Read the model definition and answer for the solid it produces. Units are mm, in the model's axes. Face numbers are marked on the shaded views. A direction names the side the tool comes from. Coordinates: 2 decimals unless noted, no trailing zeros. Loops run counter-clockwise (first coordinate to the right, second up) from the corner with the lowest first, then second, coordinate; pieces in that order, holes last. Notation, with made-up numbers: M 76,15.25 L 97,15.25 A14 ccw 97,19.25 Z; hole C 41.25,-38.75 d5. An arc over 180 degrees is marked long. One line per item, written item: value. Start each with the question number.
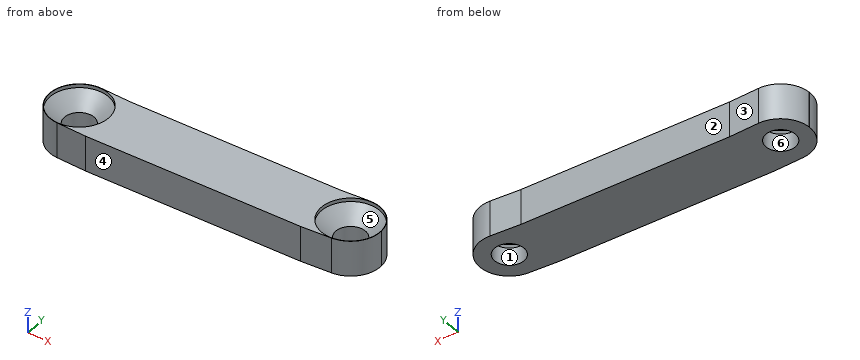
```python
from build123d import *

# Parameters (mm, degrees)
SKETCH1_R                                      = 1.25
BOSS_EXTRUDE1_DEPTH                            = 3
FILLET1_R                                      = 2.5
CSK_FOR_M2_5_FLAT_HEAD_MACHINE_SCREW2_AT_COUNT = 2
CSK_FOR_M2_5_FLAT_HEAD_MACHINE_SCREW2_AT_PITCH = 22.827023493


with BuildPart() as part:
    # Sketch1 → Boss-Extrude1 (new body)
    with BuildSketch(Plane.XY):
        Polygon((-14.040925474, -24.298454927), (-9.0477778, -24.560134708), (9.0477778, -24.560134708), (14.040925474, -24.298454927), (13.778886578, -19.298454927), (8.785738904, -19.560134708), (-8.785738904, -19.560134708), (-13.778886578, -19.298454927), align=None)
        with Locations((11.413511747, -21.93272098)):
            Circle(SKETCH1_R, mode=Mode.SUBTRACT)
        with Locations((-11.413511747, -21.93272098)):
            Circle(SKETCH1_R, mode=Mode.SUBTRACT)
    extrude(amount=BOSS_EXTRUDE1_DEPTH)

    # Fillet1
    fillet1_edges = [part.edges().sort_by_distance(p)[0] for p in [
        (-9.0477778, -24.560134708, 1.5),
        (-14.040925474, -24.298454927, 1.5),
        (-13.778886578, -19.298454927, 1.5),
        (-8.785738904, -19.560134708, 1.5),
        (8.785738904, -19.560134708, 1.5),
        (13.778886578, -19.298454927, 1.5),
        (14.040925474, -24.298454927, 1.5),
        (9.0477778, -24.560134708, 1.5),
    ]]
    fillet(fillet1_edges, radius=FILLET1_R)

    # Sketch5 → CSK for M2.5 Flat Head Machine Screw2 (revolve, cut)
    with BuildSketch(Plane(origin=(-11.413511747, -21.93272098, 3), x_dir=(0, -1, 0), z_dir=(1, 0, 0))):
        Polygon((0, 0), (0, 5.751075774), (1.25, 5), (1.25, 1.525), (2.475, 0.3), (2.475, 0), align=None)
    csk_for_m2_5_flat_head_machine_screw2 = revolve(axis=Axis((-11.413511747, -21.93272098, 9.35), (0, 0, -1)), mode=Mode.SUBTRACT)

    # CSK for M2.5 Flat Head Machine Screw2 at: CSK for M2.5 Flat Head Machine Screw2 ×2
    with Locations(*[(i * CSK_FOR_M2_5_FLAT_HEAD_MACHINE_SCREW2_AT_PITCH, 0, 0) for i in range(1, CSK_FOR_M2_5_FLAT_HEAD_MACHINE_SCREW2_AT_COUNT)]):
        add(csk_for_m2_5_flat_head_machine_screw2, mode=Mode.SUBTRACT)


solid = part.part
```
1) Section C-C (y = -22.4) is taken. Count the separate pieces of the cut face and the enclosed holes in it, then the cut area to 3 significant figures.
2) A flat-ended cylindrical pin translates along its axis: pin 1 (1.5 mm diameter, centred on x = 4.5, z = 1.5, fed in from +Y). Find the tip coordinate at first contact, or state that the pin passes through.
3) Section A-A (z = 2.1) is taken. Determine the outline of the cut face in (x, y) (3 decimals), then the cut area to 3 significant figures.
4) Consider line 1 along X through (y, z) = (-21.05, 1.65); line 2 along X through (y, z) = (-20.05, 2.6); line 3 along Y through (x, z) = (-3.5, 0.4). Determine where each line is inside the solid, lowest interval first.
5) For a pull along Y with two mould halves and no side action, classify the marked faces 3, 4, 5 and 6 as released by +Y, released by -Y, zero draft, split by the parting line, or undercut.
6) A tool of negligible diameter and unlimited length cuts with its end or side. For the marked faces 1 and 2, from which of +Z, -Z, +X, -X, +Y, -Y can it reach the whole face along a straight path? Write none if from no direction.
7) Section B-B (x = -6) is taken. Determine the outline of the cut face in (y, z).
Results found:
1. separate pieces: 3
1. enclosed holes: 0
1. area: 64.6 mm²
2. pin 1: stops at y = -19.56
3. outline: M -13.91,-21.802 A2.5 ccw -11.544,-24.429 L -9.048,-24.56 L 9.048,-24.56 L 11.544,-24.429 A2.5 ccw 13.91,-21.802 L 13.91,-21.795 A2.5 ccw 11.282,-19.429 L 8.786,-19.56 L -8.786,-19.56 L -11.282,-19.429 A2.5 ccw -13.91,-21.795 Z; hole C -11.414,-21.933 d3.75; hole C 11.414,-21.933 d3.75
3. area: 112 mm²
4. line 1: x = -13.75 to -12.53, -10.29 to 10.29, 12.53 to 13.75
4. line 2: x = -13.07 to -12.86, -9.97 to 9.97, 12.86 to 13.07
4. line 3: y = -24.56 to -19.56
5. face 3: released by +Y
5. face 4: released by -Y
5. face 5: undercut
5. face 6: undercut
6. face 1: +Z, -Z
6. face 2: +Z, -Z, +Y
7. outline: M -24.56,0 L -19.56,0 L -19.56,3 L -24.56,3 Z
